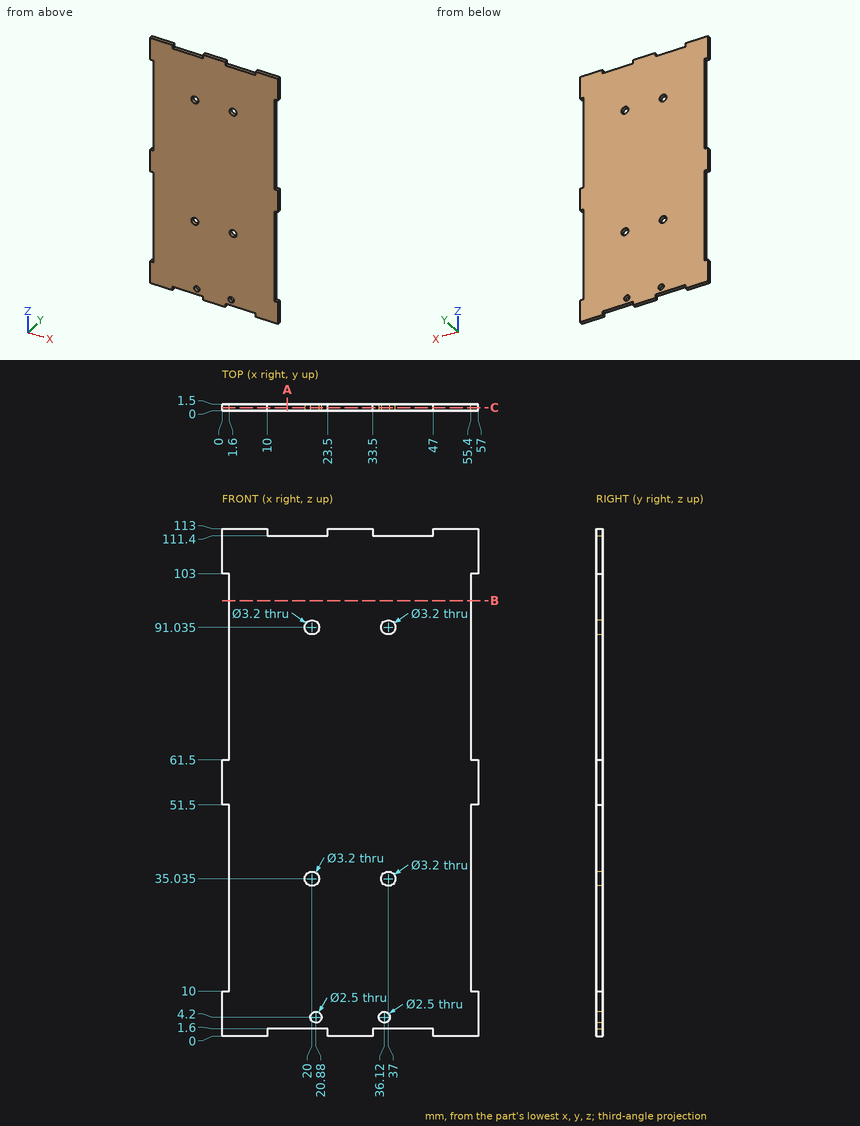
Input: dimensioned drawing with shaded views. Units: mm. Origin: part minimum x, y, z. Coordinates: 2 decimals unless noted, no trailing zeros. Order: outer loops, then holes, each group sorted by start corner. A loop starts at its lowest first (then second) coordinate and runs counter-clockwise, first axis right, second up.
1. Ray query, line 1 along X through (y, z) = (0.35, 34.5); line 2 along Z through (x, y) = (21, 0.85) (1 decimal); line 3 along Z through (x, y) = (39.5, 0.5). Return the intervals inside material, ascending.
Checked values:
line 1: x = 1.6 to 18.49, 21.51 to 35.49, 38.51 to 55.4
line 2: z = 1.6 to 3, 5.4 to 33.8, 36.3 to 89.8, 92.3 to 111.4
line 3: z = 1.6 to 111.4
2. Cut plane A-A, the plane x = 14.5. Return loops of the section in (y, z), plus the area to 3 significant figures.
Checked values:
outline: (0, 1.6) - (1.5, 1.6) - (1.5, 111.4) - (0, 111.4) - close
area: 165 mm2
3. Cut plane C-C, the plane y = 0.7. Count the separate pieces of the cut face and the enclosed holes in it, plus the area to 3 significant figures.
Checked values:
separate pieces: 1
enclosed holes: 6
area: 6,050 mm2
4. Cut plane B-B, the plane z = 97. Return loops of the section in (x, y).
Checked values:
outline: (1.6, 0) - (55.4, 0) - (55.4, 1.5) - (1.6, 1.5) - close
